Geometry check sheet. Reference: the model listing, model coordinates, mm. A direction names the side the tool comes from. Coordinates: 2 decimals unless noted, no trailing zeros. Write each loop counter-clockwise with the first axis right and the second up, starting at its lowest first coordinate (ties: lowest second). Pieces come first, ordered by that corner, then holes. Notation, with made-up numbers: M 4,63.25 L 38,63.25 A29 ccw 38,90.25 Z; hole C 27,84 d8. An arc over 180 degrees is marked long. Write each question's results on one line, items separated by ' | '.
Autodesk Inventor part; units mm, degrees
ref_plane "YZ Plane" through (0, 0, 0) normal (1, 0, 0) x (0, 1, 0)
ref_plane "XZ Plane" through (0, 0, 0) normal (0, 1, 0) x (-1, 0, 0)
ref_plane "XY Plane" through (0, 0, 0) normal (0, 0, 1) x (1, 0, 0)
ref_plane "Work Plane3" through (-1117.6, -50.8, 0) normal (0, 0, -1) x (-1, 0, 0)
sketch "Sketch1" plane through (-1117.6, -50.8, 0) normal (0, 0, -1) x (-1, 0, 0)
  line L0 (76.5714, 47.2114) -> (29.5714, 47.2114)
  line L1 (29.5714, 47.2114) -> (29.5714, 0.2114)
  line L2 (29.5714, 0.2114) -> (76.5714, 0.2114)
  line L3 (76.5714, 0.2114) -> (76.5714, 47.2114)
  circle A0 centre (70.838, 41.6003) radius 1.3139
  line L4 (74.6603, 45.4225) -> (31.3603, 45.4225)
  line L5 (31.3603, 45.4225) -> (31.3603, 2.1225)
  line L6 (31.3603, 2.1225) -> (74.6603, 2.1225)
  line L7 (74.6603, 2.1225) -> (74.6603, 45.4225)
  circle A1 centre (35.3047, 41.4781) radius 1.3139
  circle A2 centre (35.3047, 5.9448) radius 1.3139
  circle A3 centre (70.838, 5.9448) radius 1.3139
  circle A4 centre (35.3047, 5.9448) radius 3.1056
  circle A5 centre (70.838, 5.9448) radius 3.1056
  circle A6 centre (70.838, 41.6003) radius 3.1056
  circle A7 centre (35.3047, 41.4781) radius 3.1056
  line L8 (38.6492, 9.2892) -> (67.4936, 9.2892)
  line L9 (67.4936, 9.2892) -> (67.4936, 38.1337)
  line L10 (67.4936, 38.1337) -> (38.6492, 38.1337)
  line L11 (38.6492, 38.1337) -> (38.6492, 9.2892)
  point P0 (-1117.6, 50.8)
  point P1 (53.0714, 47.2114)
  point P2 (53.0714, 0.2114)
  dimension "d1" = 47
  dimension "d2" = 47
  dimension "d4" = 2.6278
  dimension "d5" = 5.7333
  dimension "d6" = 1.9111
  dimension "d7" = 1.9111
  dimension "d8" = 43.3
  dimension "d9" = 43.3
  dimension "d10" = 2.6278
  dimension "d11" = 3.8222
  dimension "d12" = 5.7333
  dimension "d13" = 5.7333
  dimension "d14" = 2.6278
  dimension "d15" = 5.7333
  dimension "d16" = 5.7333
  dimension "d17" = 2.6278
  dimension "d18" = 5.7333
  dimension "d19" = 3.8222
  dimension "d20" = 6.2111
  dimension "d21" = 6.2111
  dimension "d22" = 6.2111
  dimension "d23" = 6.2111
  dimension "d24" = 9.0778
  dimension "d25" = 9.0778
  dimension "d26" = 9.0778
  dimension "d27" = 9.0778
extrude "Extrusion3" add sketch "Sketch1" along normal blind 8 contours L3 L2 L1 L0
extrude "Extrusion6" add sketch "Sketch1" along normal blind 10 contours A0 | A1 | A2 | A3
extrude "Extrusion7" add sketch "Sketch1" along normal blind 4 contours A2 | A4 | A5 | A6 | A7
extrude "Extrusion8" add sketch "Sketch1" against normal blind 3 contours L3 L2 L1 L0 | A0 | L7 L6 L5 L4 | A1 | A2 | A3 | A4 | A5 | A6 | A7
fillet "Fillet5" radius 10 4 edges at (-1156.2492, -12.6663, 1.5) (-1185.0936, -12.6663, 1.5) (-1185.0936, -41.5108, 1.5) (-1156.2492, -41.5108, 1.5)
fillet "Fillet6" radius 2 4 edges at (-1194.1714, -3.5886, -2.5) (-1147.1714, -3.5886, -2.5) (-1194.1714, -50.5886, -2.5) (-1147.1714, -50.5886, -2.5)
properties part number "mnt298bracket"
Q1. Sectioned sample at B-B on z = -4.75. Record the cut outline in (x, y), and give its area (3 significant figures).
Geometry check:
outline: M -1194.17,-48.59 A2 ccw -1192.17,-50.59 L -1149.17,-50.59 A2 ccw -1147.17,-48.59 L -1147.17,-5.59 A2 ccw -1149.17,-3.59 L -1192.17,-3.59 A2 ccw -1194.17,-5.59 Z; C -1188.44,-44.86 d2.63; C -1188.44,-9.2 d2.63; C -1152.9,-44.86 d2.63; C -1152.9,-9.32 d2.63; hole M -1192.26,-48.68 L -1148.96,-48.68 L -1148.96,-5.38 L -1192.26,-5.38 Z | area: 352 mm2
Q2. Sectioned sample at C-C on y = -24. Record the cut outline in (x, z).
Geometry check:
outline: M -1194.17,-8 L -1192.26,-8 L -1192.26,0 L -1185.09,0 L -1185.09,3 L -1194.17,3 Z; M -1156.25,0 L -1148.96,0 L -1148.96,-8 L -1147.17,-8 L -1147.17,3 L -1156.25,3 Z
Q3. Scan lines: probe 1 along Y at (x, z) = (-1166, -1); probe 2 along Y at (x, z) = (-1167, 1.5); probe 3 along Y at (x, z) = (-1152, -0.25). Record each from-to range of solid material in increasing order.
Geometry check:
probe 1: y = -50.59 to -48.68, -5.38 to -3.59 | probe 2: y = -50.59 to -41.51, -12.67 to -3.59 | probe 3: y = -50.59 to -48.68, -47.83 to -41.88, -12.29 to -6.35, -5.38 to -3.59
Q4. Sectioned sample at A-A on z = 2. Record the cut outline in (x, y).
Geometry check:
outline: M -1194.17,-48.59 A2 ccw -1192.17,-50.59 L -1149.17,-50.59 A2 ccw -1147.17,-48.59 L -1147.17,-5.59 A2 ccw -1149.17,-3.59 L -1192.17,-3.59 A2 ccw -1194.17,-5.59 Z; hole M -1185.09,-31.51 A10 ccw -1175.09,-41.51 L -1166.25,-41.51 A10 ccw -1156.25,-31.51 L -1156.25,-22.67 A10 ccw -1166.25,-12.67 L -1175.09,-12.67 A10 ccw -1185.09,-22.67 Z
Q5. Mould release check, pull along Y, two halves, no side actions. Record for faces 1 (the cylindrical face through (-1182.242, -38.504, 1.521)), 2 (the flat face through (-1153, -45, -10)), 3 (the cylindrical face through (-1193.6, -49.99, -2.42)): pulls with the +Y half, pulls with the -Y half, needs draft (parallel to the pull), parting line crosses it, or undercut.
Geometry check:
face 1: undercut | face 2: needs draft | face 3: pulls with the -Y half
Q6. Sectioned sample at D-D on x = -1178. Record the cut outline in (y, z).
Geometry check:
outline: M -50.59,-8 L -48.68,-8 L -48.68,0 L -41.08,0 L -41.08,3 L -50.59,3 Z; M -13.1,0 L -5.38,0 L -5.38,-8 L -3.59,-8 L -3.59,3 L -13.1,3 Z
Q7. Access from +Z, -Z, +X, -X, +Y, -Y to the whole of each face (thin tool, end or side, straight path). Record for faces 4 (the cylindrical face through (-1191.31, -43.67, -1.97)), 5 (the cylindrical face through (-1147.77, -4.16, -2.58)), 6 (the flat face through (-1171, -12.666, 1)).
Geometry check:
face 4: -Z | face 5: +Z, -Z, +X, +Y | face 6: +Z, -Z
Q8. Depth check by flat-ended pin: P1, Ø1.5, axis at x = -1164.5, y = -43.5, coming from the -Z side; P2, Ø13, axis at x = -1169, y = -28, coming from the -Z side. Enter the tip coordinate at first touch or a pass-through.
Geometry check:
P1: stops at z = 0 | P2: passes through
